Geometry check sheet. Reference: drawing and pictorial views, mm from the part's lowest x, y, z. A direction names the side the tool comes from. Give positions to 0.01 mm unless a question says otherwise; leave off trailing zeros. Order: outer loops, then holes, each group sorted by start corner. A loop starts at its lowest first (then second) coordinate and runs counter-clockwise, first axis right, second up. Notation, with made-up numbers: (39, 56.25) - (73, 56.25) arc R9 ccw to (73, 69.25) - close; hole circle Ø6 at (23, -10.5). An arc over 180 degrees is marked (long way). Answer as a JSON object with one key per item and string values.
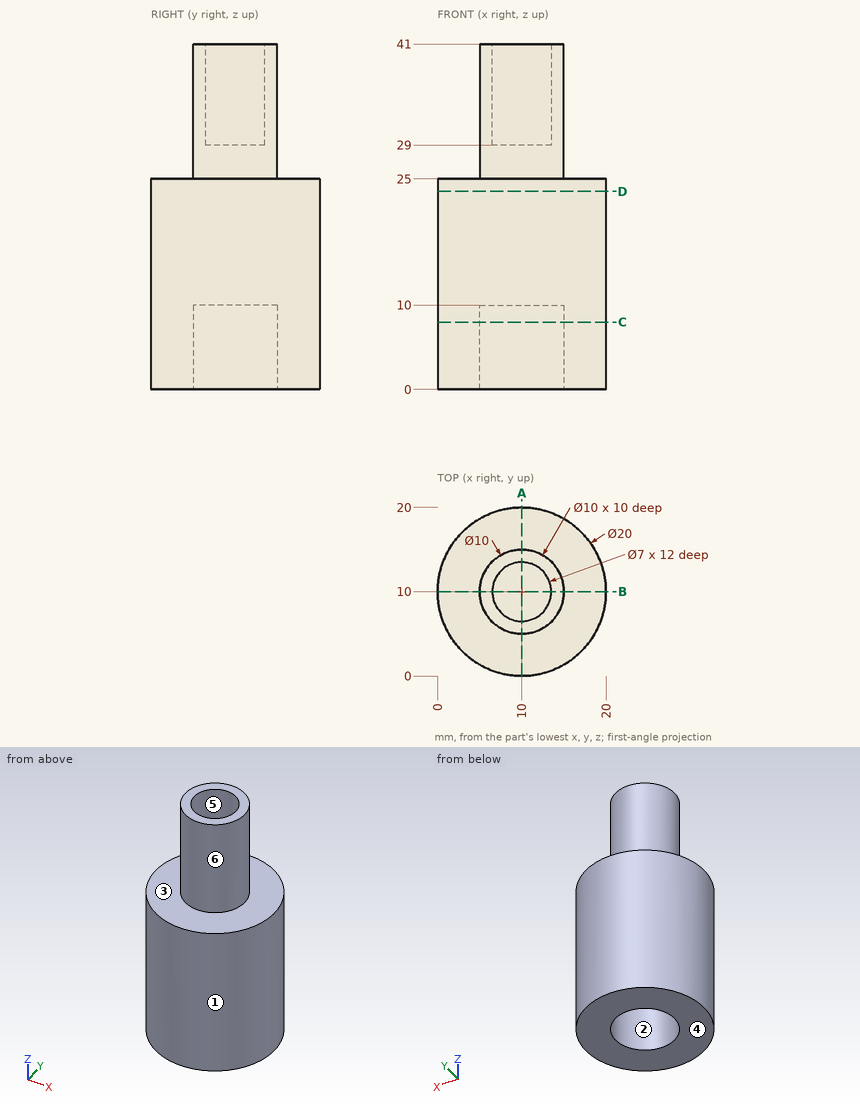
(1) Material ranges on line 1 along Y through (x, z) = (10, 6); line 2 along Y through (x, z) = (10, 33.25); line 3 along Z through (x, y) = (13.25, 2), recorded low to high. Write a range as [from, to].
Computed values:
{"line 1": "y = [0, 5], [15, 20]", "line 2": "y = [5, 6.5], [13.5, 15]", "line 3": "z = [0, 25]"}
(2) Section check A-A (x = 10). Record the cut outline in (y, z), then the cut area to 3 significant figures.
Computed values:
{"outline": "(0, 0) - (5, 0) - (5, 10) - (15, 10) - (15, 0) - (20, 0) - (20, 25) - (15, 25) - (15, 41) - (13.5, 41) - (13.5, 29) - (6.5, 29) - (6.5, 41) - (5, 41) - (5, 25) - (0, 25) - close", "area": "476 mm²"}
(3) Gauge pin test, flat ends, axial feed: pin 1 Ø4 at (x, y) = (10, 10) entering from +Z; pin 2 Ø6 at (x, y) = (5.5, 2.5) entering from +Z; pin 3 Ø2 at (y, z) = (11.5, 10.5) entering from +X. Record the tip position at first contact, or that the pin passes through.
Computed values:
{"pin 1": "stops at z = 29", "pin 2": "stops at z = 25", "pin 3": "stops at x = 19.99"}
(4) Section check C-C (z = 8). Record the cut outline in (x, y).
Computed values:
{"outline": "circle Ø20 at (10, 10); hole circle Ø10 at (10, 10)"}
(5) Access from +Z, -Z, +X, -X, +Y, -Y to the whole of each face (thin tool, end or side, straight path). Record for the marked faces 1, 2 and 3.
Computed values:
{"face 1": "+Z, -Z", "face 2": "-Z", "face 3": "+Z"}
(6) Section check D-D (z = 23.5). Record the cut outline in (x, y), then the cut area to 3 significant figures.
Computed values:
{"outline": "circle Ø20 at (10, 10)", "area": "314 mm²"}
(7) Release check for a two-part mould opening along X. For the marked faces 4, 5 and 6 record: pulls with the +X half, pulls with the -X half, needs draft (parallel to the pull), parting line crosses it, or undercut.
Computed values:
{"face 4": "needs draft", "face 5": "undercut", "face 6": "parting line crosses it"}
